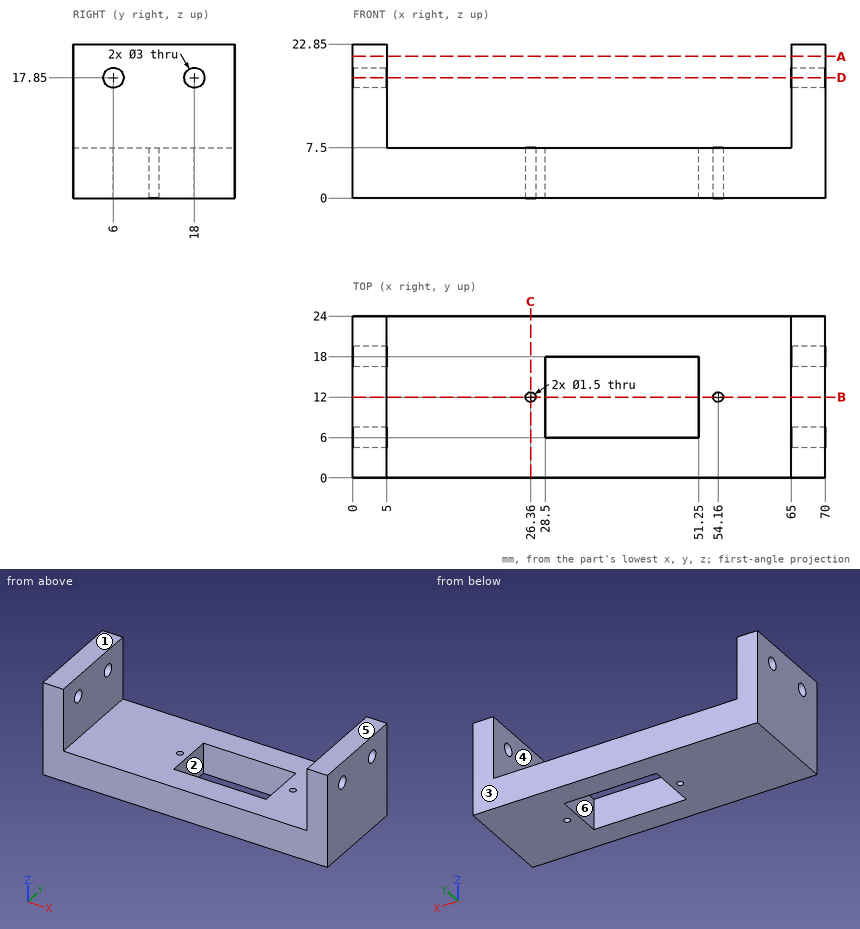
Study the drawing (mm; zero at the part's minimum x, y, z) and answer. A direction names the side the tool comes from. Coordinates: 2 decimals unless noted, no trailing zeros. Loops run counter-clockwise (first coordinate to the right, second up) from the corner with the lowest first, then second, coordinate; pieces in that order, holes last. Notation, with made-up numbers: (22.5, -22) -> (51.5, -22) arc R19 cw to (51.5, -11) -> close; hole circle Ø2 at (23, 65). An arc over 180 degrees is marked (long way). Write item = value, one per line. Start each with the question number.
1) The mould has two halves that part along Y. Classify the marked faces 1, 2 and 3: pulls with the +Y half, pulls with the -Y half, needs draft (parallel to the pull), parting line crosses it, or undercut.
2) The part is cut by section C-C, the plane x = 26.36. Determine the outline of the cut face in (y, z).
3) The part is cut by section A-A, the plane z = 21. Determine the outline of the cut face in (x, y), plus the area to 3 significant figures.
4) Given P1, Ø4, axis at y = 9.5, z = 18, coming from the -X side; P2, Ø3, axis at x = 16, y = 21.5, coming from the +Z side, each flat-ended and moving along its own axis, determine where each tip first touches the part or whether it passes through.
5) The part is cut by section B-B, the plane y = 12. Determine the outline of the cut face in (x, z).
6) Find the intervals of material crossed by L1, parallel to Y at x = 68.7, z = 17.85; L2, parallel to X at y = 7, z = 15; L3, parallel to Y at x = 26.36, z = 4, in increasing order. Write a range as from..to.
7) The part is cut by section D-D, the plane z = 17.85. Determine the outline of the cut face in (x, y).
8) For the marked faces 4, 5 and 6, determine the directions among +Z, -Z, +X, -X, +Y, -Y from which every point of the face is accessible in a straight line to the end or side of a thin tool.
Result:
q1.face_1 = needs draft
q1.face_2 = undercut
q1.face_3 = pulls with the +Y half
q2.outline = (0, 0) -> (11.25, 0) -> (11.25, 7.5) -> (0, 7.5) -> close; (12.75, 0) -> (24, 0) -> (24, 7.5) -> (12.75, 7.5) -> close
q3.outline = (0, 0) -> (5, 0) -> (5, 24) -> (0, 24) -> close; (65, 0) -> (70, 0) -> (70, 24) -> (65, 24) -> close
q3.area = 240 mm²
q4.P1 = 0
q4.P2 = 7.5
q5.outline = (0, 0) -> (25.61, 0) -> (25.61, 7.5) -> (5, 7.5) -> (5, 22.85) -> (0, 22.85) -> close; (27.11, 0) -> (28.5, 0) -> (28.5, 7.5) -> (27.11, 7.5) -> close; (51.25, 0) -> (53.41, 0) -> (53.41, 7.5) -> (51.25, 7.5) -> close; (54.91, 0) -> (70, 0) -> (70, 22.85) -> (65, 22.85) -> (65, 7.5) -> (54.91, 7.5) -> close
q6.L1 = 0..4.5, 7.5..16.5, 19.5..24
q6.L2 = 0..5, 65..70
q6.L3 = 0..11.25, 12.75..24
q7.outline = (0, 0) -> (5, 0) -> (5, 4.5) -> (0, 4.5) -> close; (0, 7.5) -> (5, 7.5) -> (5, 16.5) -> (0, 16.5) -> close; (0, 19.5) -> (5, 19.5) -> (5, 24) -> (0, 24) -> close; (65, 0) -> (70, 0) -> (70, 4.5) -> (65, 4.5) -> close; (65, 7.5) -> (70, 7.5) -> (70, 16.5) -> (65, 16.5) -> close; (65, 19.5) -> (70, 19.5) -> (70, 24) -> (65, 24) -> close
q8.face_4 = +Z, +Y, -Y
q8.face_5 = +Z, +X, -X, +Y, -Y
q8.face_6 = +Z, -Z
